```python
from build123d import *

# Parameters (mm, degrees)
SKETCH1_W           = 7.5
SKETCH1_H           = 20
BOSS_EXTRUDE1_DEPTH = 2
SKETCH2_W           = 5
SKETCH2_H           = 5
BOSS_EXTRUDE2_DEPTH = 4
SKETCH3_W           = 5
SKETCH3_H           = 72.5
BOSS_EXTRUDE3_DEPTH = 2
SKETCH4_W           = 2
SKETCH4_H           = 40
BOSS_EXTRUDE4_DEPTH = 40
FILLET1_R           = 1
FILLET2_R           = 1


with BuildPart() as part:
    # Sketch1 → Boss-Extrude1 (new body)
    with BuildSketch(Plane.XY):
        Rectangle(SKETCH1_W, SKETCH1_H)
    extrude(amount=BOSS_EXTRUDE1_DEPTH)

    # Sketch2 → Boss-Extrude2 (add)
    with BuildSketch(Plane(origin=(0, 0, 0), x_dir=(-1, 0, 0), z_dir=(0, 0, -1))):
        Rectangle(SKETCH2_W, SKETCH2_H)
    extrude(amount=BOSS_EXTRUDE2_DEPTH)

    # Sketch3 → Boss-Extrude3 (add)
    with BuildSketch(Plane(origin=(0, 0, -4), x_dir=(-1, 0, 0), z_dir=(0, 0, -1))):
        with Locations((0, 36.25)):
            Rectangle(SKETCH3_W, SKETCH3_H)
    extrude(amount=BOSS_EXTRUDE3_DEPTH)

    # Sketch4 → Boss-Extrude4 (add)
    with BuildSketch(Plane.XY.offset(-4)):
        with Locations((0, 52.5)):
            Rectangle(SKETCH4_W, SKETCH4_H)
    extrude(amount=BOSS_EXTRUDE4_DEPTH)

    # Fillet1
    fillet1_edges = [part.edges().sort_by_distance(p)[0] for p in [
        (0, 0, -4),
    ]]
    fillet(fillet1_edges, radius=FILLET1_R)

    # Fillet2
    fillet2_edges = [part.edges().sort_by_distance(p)[0] for p in [
        (-1, 52.5, -4),
        (0, 32.5, -4),
        (1, 52.5, -4),
    ]]
    fillet(fillet2_edges, radius=FILLET2_R)


solid = part.part
```
Verification items for the finished model (mm, model axes). A direction names the side the tool comes from. Coordinates: 2 decimals unless noted, no trailing zeros. Write each loop counter-clockwise with the first axis right and the second up, starting at its lowest first coordinate (ties: lowest second). Pieces come first, ordered by that corner, then holes. Notation, with made-up numbers: M 50,58 L 108,58 A21 cw 108,96 Z; hole C -6.75,-19.5 d9. An arc over 180 degrees is marked long. Answer as a JSON object with one key per item and string values. Group by question number.
(1) Gauge pin test, flat ends, axial feed: pin 1 (1.5 mm diameter, centred on x = -1, y = 25, fed in from +Z); pin 2 (0.8 mm diameter, centred on x = -0.5, y = -2, fed in from -Z); pin 3 (11.5 mm diameter, centred on y = 52.5, z = 16, fed in from -X). Record the tip position at first contact, or that the pin passes through.
(2) Cross-section at C-C, the plane y = 27.5. Record the cut outline in (x, z), and give its area (3 significant figures).
(3) Material ranges on line 1 (Y direction, x = -0.25, z = -3); line 2 (Z direction, x = -2, y = 7); line 3 (Y direction, x = 0, z = 18.5), recorded low to high.
(4) Cross-section at B-B, the plane z = 22. Record the cut outline in (x, y), and give its area (3 significant figures).
(5) Tool access check on faces 5 (the face through (0, 0, 2)), 6 (the face through (-2.5, 26.1, -4.3)), 7 (the face through (0, -2.5, -2)), 8 (the face through (2.5, 26.1, -4.3)), 9 (the face through (0, 10, 1)). Record the directions out of +Z, -Z, +X, -X, +Y, -Y that give a thin tool (end or side, any length) a straight path to the whole face; none if there is none.
(6) Release check for a two-part mould opening along Y. For faces 1 (the face through (0, -10, 1)), 2 (the face through (0, 72.5, 14)), 3 (the face through (0, -2, -4)), 4 (the face through (0, 2.5, -2)) record: +Y half, -Y half, draft (parallel to the pull), parting line (faces both ways), or undercut.
(7) Cross-section at A-A, the plane y = 39.5. Record the cut outline in (x, z).
Reply:
{
 "1": {"pin 1": "z = -4", "pin 2": "z = -4", "pin 3": "x = -1"},
 "2": {"outline": "M -2.5,-6 L 2.5,-6 L 2.5,-4 L -2.5,-4 Z", "area": "10.0 mm²"},
 "3": {"line 1": "-2.5 to 2.5, 32.5 to 72.5", "line 2": "-6 to -4, 0 to 2", "line 3": "32.5 to 72.5"},
 "4": {"outline": "M -1,32.5 L 1,32.5 L 1,72.5 L -1,72.5 Z", "area": "80.0 mm²"},
 "5": {"face 5": "+Z, +X, -X, -Y", "face 6": "-Z, -X, +Y, -Y", "face 7": "-Z, +X, -X, -Y", "face 8": "-Z, +X, +Y, -Y", "face 9": "+Z, +X, -X"},
 "6": {"face 1": "-Y half", "face 2": "+Y half", "face 3": "draft", "face 4": "undercut"},
 "7": {"outline": "M -2.5,-6 L 2.5,-6 L 2.5,-4 L 2,-4 A1 cw 1,-3 L 1,36 L -1,36 L -1,-3 A1 cw -2,-4 L -2.5,-4 Z"}
}
